```python
from build123d import *

# Parameters (mm, degrees)
SKETCH1_R                  = 6.5
BOSS_EXTRUDE1_DEPTH        = 5
SKETCH2_W                  = 14
SKETCH2_H                  = 5
BOSS_EXTRUDE2_DEPTH        = 50
SKETCH3_R                  = 2.75
CUT_EXTRUDE1_DEPTH         = 115
FILLET2_R                  = 10
CUT_EXTRUDE2_DEPTH         = 74.994932259
CIRPATTERN1_COUNT          = 4
BOSS_EXTRUDE5_START        = -5
BOSS_EXTRUDE5_DEPTH        = 5
FILLET5_R                  = 10
FILLET6_R                  = 10
FLATTEN_BENDS6_START       = -45
FLATTEN_BENDS6_OUTLINE_W   = 14
FLATTEN_BENDS6_OUTLINE_H   = 5
FLATTEN_BENDS6_DEPTH       = 45
FLATTEN_BENDS6_2_DEPTH     = 5
FLATTEN_BENDS6_3_OUTLINE_W = 14
FLATTEN_BENDS6_3_OUTLINE_H = 43.610839391
FLATTEN_BENDS6_3_OUTLINE_R = 2.75
FLATTEN_BENDS6_3_DEPTH     = 5
PROCESS_BENDS6_START       = -94.110839391
PROCESS_BENDS6_OUTLINE_W   = 14
PROCESS_BENDS6_OUTLINE_H   = 5
PROCESS_BENDS6_DEPTH       = 43.610839391
PROCESS_BENDS6_START_2     = 50.5
PROCESS_BENDS6_2_OUTLINE_W = 14
PROCESS_BENDS6_2_OUTLINE_H = 5
PROCESS_BENDS6_2_DEPTH     = 43.610839391
PROCESS_BENDS6_START_3     = -49.958579692
PROCESS_BENDS6_3_OUTLINE_W = 14
PROCESS_BENDS6_3_OUTLINE_H = 45
PROCESS_BENDS6_3_OUTLINE_R = 2.75
PROCESS_BENDS6_3_DEPTH     = 4.458579692
PROCESS_BENDS6_START_4     = 45.5
PROCESS_BENDS6_4_OUTLINE_W = 14
PROCESS_BENDS6_4_OUTLINE_H = 45
PROCESS_BENDS6_4_OUTLINE_R = 2.75
PROCESS_BENDS6_4_DEPTH     = 4.394100308
PROCESS_BENDS6_START_5     = 44.7634
PROCESS_BENDS6_5_OUTLINE_W = 14
PROCESS_BENDS6_5_OUTLINE_H = 45
PROCESS_BENDS6_5_OUTLINE_R = 2.75
PROCESS_BENDS6_5_DEPTH     = 5.7366
PROCESS_BENDS6_START_6     = -50.5
PROCESS_BENDS6_6_OUTLINE_W = 14
PROCESS_BENDS6_6_OUTLINE_H = 45
PROCESS_BENDS6_6_OUTLINE_R = 2.75
PROCESS_BENDS6_6_DEPTH     = 5.7366
PROCESS_BENDS6_START_7     = 5
PROCESS_BENDS6_7_DEPTH     = 14


with BuildPart() as part:
    # Sketch1 → Boss-Extrude1 (new body)
    with BuildSketch(Plane.XY):
        with BuildLine():
            Line((7.22970639, 29.115826375), (7.22970639, 45.5))
            Line((7.22970639, 45.5), (-7.22970639, 45.5))
            Line((-7.22970639, 45.5), (-7.22970639, 29.115826375))
            ThreePointArc((-7.22970639, 29.115826375), (-30, 0), (-7.22970639, -29.115826375))
            Line((-7.22970639, -29.115826375), (-7.22970639, -45.5))
            Line((-7.22970639, -45.5), (7.22970639, -45.5))
            Line((7.22970639, -45.5), (7.22970639, -29.115826375))
            ThreePointArc((7.22970639, -29.115826375), (30, 0), (7.22970639, 29.115826375))
        make_face()
        Circle(SKETCH1_R, mode=Mode.SUBTRACT)
    extrude(amount=BOSS_EXTRUDE1_DEPTH)

    # Sketch2 → Boss-Extrude2 (add)
    with BuildSketch(Plane.XY.offset(5)):
        with Locations((12, 48)):
            Rectangle(SKETCH2_W, SKETCH2_H)
        with Locations((12, -48)):
            Rectangle(SKETCH2_W, SKETCH2_H)
    extrude(amount=-BOSS_EXTRUDE2_DEPTH)

    # Sketch3 → Cut-Extrude1 (cut)
    with BuildSketch(Plane(origin=(0, 50.5, 0), x_dir=(1, 0, 0), z_dir=(0, 1, 0))):
        with Locations(Location((12, 40, 0), (0, 0, 270))):
            Circle(SKETCH3_R)
        with Locations(Location((12, 25, 0), (0, 0, 270))):
            Circle(SKETCH3_R)
    extrude(amount=-CUT_EXTRUDE1_DEPTH, mode=Mode.SUBTRACT)

    # Fillet2
    fillet2_edges = [part.edges().sort_by_distance(p)[0] for p in [
        (7.22970639, -29.115826375, 2.5),
        (-7.22970639, -29.115826375, 2.5),
        (-7.22970639, 29.115826375, 2.5),
        (7.22970639, 29.115826375, 2.5),
    ]]
    fillet(fillet2_edges, radius=FILLET2_R)

    # Sketch4 → Cut-Extrude2 (cut, through all)
    with BuildSketch(Plane(origin=(0, 0, 0), x_dir=(-1, 0, 0), z_dir=(0, 0, -1))):
        with BuildLine():
            Line((-2.993018736, 21.795454545), (-1.496509368, -0.102272727))
            ThreePointArc((-1.496509368, -0.102272727), (0, -1.5), (1.496509368, -0.102272727))
            Line((1.496509368, -0.102272727), (2.993018736, 21.795454545))
            ThreePointArc((2.993018736, 21.795454545), (0, 25), (-2.993018736, 21.795454545))
        make_face()
    cut_extrude2 = extrude(amount=-CUT_EXTRUDE2_DEPTH, mode=Mode.SUBTRACT)

    # CirPattern1: Cut-Extrude2 ×4 about axis
    cirpattern1_axis = Axis((0, 0, 0), (0, 0, 1))
    for i in range(1, CIRPATTERN1_COUNT):
        add(cut_extrude2.rotate(cirpattern1_axis, i * 360 / CIRPATTERN1_COUNT), mode=Mode.SUBTRACT)

    # Sketch41 → Boss-Extrude5 (add)
    with BuildSketch(Plane.XY.offset(5).offset(BOSS_EXTRUDE5_START)):
        with BuildLine():
            Line((7.22970639, 45.5), (19, 45.5))
            Line((19, 45.5), (19, 23.216373532))
            ThreePointArc((19, 23.216373532), (16.077275199, 25.32826923), (12.922279793, 27.074243941))
            ThreePointArc((12.922279793, 27.074243941), (8.771743693, 30.763931751), (7.22970639, 36.098991921))
            Line((7.22970639, 36.098991921), (7.22970639, 45.5))
        make_face()
        with BuildLine():
            Line((19, -45.5), (7.22970639, -45.5))
            Line((7.22970639, -45.5), (7.22970639, -36.098991921))
            ThreePointArc((7.22970639, -36.098991921), (8.771743693, -30.763931751), (12.922279793, -27.074243941))
            ThreePointArc((12.922279793, -27.074243941), (16.077275199, -25.32826923), (19, -23.216373532))
            Line((19, -23.216373532), (19, -45.5))
        make_face()
    extrude(amount=BOSS_EXTRUDE5_DEPTH)

    # Fillet5
    fillet5_edges = [part.edges().sort_by_distance(p)[0] for p in [
        (19, 23.216373532, 2.5),
        (19, -23.216373532, 2.5),
    ]]
    fillet(fillet5_edges, radius=FILLET5_R)

    # Fillet6
    fillet6_edges = [part.edges().sort_by_distance(p)[0] for p in [
        (-7.22970639, 45.5, 2.5),
        (-7.22970639, -45.5, 2.5),
    ]]
    fillet(fillet6_edges, radius=FILLET6_R)

    # Flatten-Bends6: read off the stored shape, not the designer's step
    # Flatten-Bends6 outline → Flatten-Bends6 (cut)
    with BuildSketch(Plane.XY.offset(FLATTEN_BENDS6_START)):
        with Locations((12, 48)):
            Rectangle(FLATTEN_BENDS6_OUTLINE_W, FLATTEN_BENDS6_OUTLINE_H)
        with Locations((12, -48)):
            Rectangle(FLATTEN_BENDS6_OUTLINE_W, FLATTEN_BENDS6_OUTLINE_H)
    extrude(amount=FLATTEN_BENDS6_DEPTH, mode=Mode.SUBTRACT)

    # Flatten-Bends6 2 outline → Flatten-Bends6 2 (cut)
    with BuildSketch(Plane.XY):
        with BuildLine():
            Line((5, 42.2634), (5, 45.5))
            Line((5, 45.5), (2.761321814, 45.5))
            ThreePointArc((2.761321814, 45.5), (2.63064975, 45.499146204), (2.5, 45.496584962))
            Line((2.5, 45.496584962), (2.5, 42.2634))
            Line((2.5, 42.2634), (5, 42.2634))
        make_face()
        with BuildLine():
            Line((5, -45.5), (5, -42.2634))
            Line((5, -42.2634), (2.5, -42.2634))
            Line((2.5, -42.2634), (2.5, -45.496584962))
            ThreePointArc((2.5, -45.496584962), (2.63064975, -45.499146204), (2.761321814, -45.5))
            Line((2.761321814, -45.5), (5, -45.5))
        make_face()
    extrude(amount=FLATTEN_BENDS6_2_DEPTH, mode=Mode.SUBTRACT)

    # Flatten-Bends6 3 outline → Flatten-Bends6 3 (add)
    # profile 1 of 2: a face of its own
    with BuildSketch(Plane.XY):
        with Locations((12, 72.305419696)):
            Rectangle(FLATTEN_BENDS6_3_OUTLINE_W, FLATTEN_BENDS6_3_OUTLINE_H)
        with Locations((12, 74.110839391)):
            Circle(FLATTEN_BENDS6_3_OUTLINE_R, mode=Mode.SUBTRACT)
        with Locations((12, 89.110839391)):
            Circle(FLATTEN_BENDS6_3_OUTLINE_R, mode=Mode.SUBTRACT)
    # profile 2 of 2: a face of its own
    with BuildSketch(Plane.XY):
        with Locations((12, -72.305419696)):
            Rectangle(FLATTEN_BENDS6_3_OUTLINE_W, FLATTEN_BENDS6_3_OUTLINE_H)
        with Locations((12, -89.110839391)):
            Circle(FLATTEN_BENDS6_3_OUTLINE_R, mode=Mode.SUBTRACT)
        with Locations((12, -74.110839391)):
            Circle(FLATTEN_BENDS6_3_OUTLINE_R, mode=Mode.SUBTRACT)
    extrude(amount=FLATTEN_BENDS6_3_DEPTH)

    # Process-Bends6: read off the stored shape, not the designer's step
    # Process-Bends6 outline → Process-Bends6 (cut)
    with BuildSketch(Plane(origin=(0, 0, 0), x_dir=(1, 0, 0), z_dir=(0, 1, 0)).offset(PROCESS_BENDS6_START)):
        with Locations((12, -2.5)):
            Rectangle(PROCESS_BENDS6_OUTLINE_W, PROCESS_BENDS6_OUTLINE_H)
    extrude(amount=PROCESS_BENDS6_DEPTH, mode=Mode.SUBTRACT)

    # Process-Bends6 2 outline → Process-Bends6 2 (cut)
    with BuildSketch(Plane(origin=(0, 0, 0), x_dir=(1, 0, 0), z_dir=(0, 1, 0)).offset(PROCESS_BENDS6_START_2)):
        with Locations((12, -2.5)):
            Rectangle(PROCESS_BENDS6_2_OUTLINE_W, PROCESS_BENDS6_2_OUTLINE_H)
    extrude(amount=PROCESS_BENDS6_2_DEPTH, mode=Mode.SUBTRACT)

    # Process-Bends6 3 outline → Process-Bends6 3 (add)
    with BuildSketch(Plane(origin=(0, 0, 0), x_dir=(1, 0, 0), z_dir=(0, 1, 0)).offset(PROCESS_BENDS6_START_3)):
        with Locations((12, 22.5)):
            Rectangle(PROCESS_BENDS6_3_OUTLINE_W, PROCESS_BENDS6_3_OUTLINE_H)
        with Locations((12, 25)):
            Circle(PROCESS_BENDS6_3_OUTLINE_R, mode=Mode.SUBTRACT)
        with Locations((12, 40)):
            Circle(PROCESS_BENDS6_3_OUTLINE_R, mode=Mode.SUBTRACT)
    extrude(amount=PROCESS_BENDS6_3_DEPTH)

    # Process-Bends6 4 outline → Process-Bends6 4 (add)
    with BuildSketch(Plane(origin=(0, 0, 0), x_dir=(1, 0, 0), z_dir=(0, 1, 0)).offset(PROCESS_BENDS6_START_4)):
        with Locations((12, 22.5)):
            Rectangle(PROCESS_BENDS6_4_OUTLINE_W, PROCESS_BENDS6_4_OUTLINE_H)
        with Locations((12, 25)):
            Circle(PROCESS_BENDS6_4_OUTLINE_R, mode=Mode.SUBTRACT)
        with Locations((12, 40)):
            Circle(PROCESS_BENDS6_4_OUTLINE_R, mode=Mode.SUBTRACT)
    extrude(amount=PROCESS_BENDS6_4_DEPTH)

    # Process-Bends6 5 outline → Process-Bends6 5 (add)
    with BuildSketch(Plane(origin=(0, 0, 0), x_dir=(1, 0, 0), z_dir=(0, 1, 0)).offset(PROCESS_BENDS6_START_5)):
        with Locations((12, 22.5)):
            Rectangle(PROCESS_BENDS6_5_OUTLINE_W, PROCESS_BENDS6_5_OUTLINE_H)
        with Locations((12, 25)):
            Circle(PROCESS_BENDS6_5_OUTLINE_R, mode=Mode.SUBTRACT)
        with Locations((12, 40)):
            Circle(PROCESS_BENDS6_5_OUTLINE_R, mode=Mode.SUBTRACT)
    extrude(amount=PROCESS_BENDS6_5_DEPTH)

    # Process-Bends6 6 outline → Process-Bends6 6 (add)
    with BuildSketch(Plane(origin=(0, 0, 0), x_dir=(1, 0, 0), z_dir=(0, 1, 0)).offset(PROCESS_BENDS6_START_6)):
        with Locations((12, 22.5)):
            Rectangle(PROCESS_BENDS6_6_OUTLINE_W, PROCESS_BENDS6_6_OUTLINE_H)
        with Locations((12, 25)):
            Circle(PROCESS_BENDS6_6_OUTLINE_R, mode=Mode.SUBTRACT)
        with Locations((12, 40)):
            Circle(PROCESS_BENDS6_6_OUTLINE_R, mode=Mode.SUBTRACT)
    extrude(amount=PROCESS_BENDS6_6_DEPTH)

    # Process-Bends6 7 outline → Process-Bends6 7 (cut)
    with BuildSketch(Plane.YZ.offset(PROCESS_BENDS6_START_7)):
        with BuildLine():
            Line((-45.5, -0.7366), (-45.5, -45))
            Line((-45.5, -45), (-44.7634, -45))
            Line((-44.7634, -45), (-44.7634, 0))
            ThreePointArc((-44.7634, 0), (-45.284254855, -0.215745145), (-45.5, -0.7366))
        make_face()
        with BuildLine():
            ThreePointArc((-50.5, -0.7366), (-48.819788761, 3.319788761), (-44.7634, 5))
            Line((-44.7634, 5), (-50.5, 5))
            Line((-50.5, 5), (-50.5, -0.7366))
        make_face()
        with BuildLine():
            ThreePointArc((44.7634, 5), (48.819788761, 3.319788761), (50.5, -0.7366))
            Line((50.5, -0.7366), (50.5, 5))
            Line((50.5, 5), (44.7634, 5))
        make_face()
        with BuildLine():
            Line((45.5, -45), (45.5, -0.7366))
            ThreePointArc((45.5, -0.7366), (45.284254855, -0.215745145), (44.7634, 0))
            Line((44.7634, 0), (44.7634, -45))
            Line((44.7634, -45), (45.5, -45))
        make_face()
    extrude(amount=PROCESS_BENDS6_7_DEPTH, mode=Mode.SUBTRACT)


solid = part.part
```
Input: part model. Units: mm. Frame: model coordinates. A direction names the side the tool comes from. Coordinates: 2 decimals unless noted, no trailing zeros. Write each loop counter-clockwise with the first axis right and the second up, starting at its lowest first coordinate (ties: lowest second). Pieces come first, ordered by that corner, then holes. Notation, with made-up numbers: (-10, 65) -> (-3, 65) arc R3 ccw to (-3, 69) -> close; hole circle Ø3 at (52.5, -4.75). An arc over 180 degrees is marked (long way). Write each question's results on one line, items separated by ' | '.
Item 1: Set-up query: faces 5 (the flat face through (2.5, -44, 2)), 6 (the flat face through (14.111, -2.468, 2.465)), 7 (the flat face through (10.3, -45.5, -22.6)). Return all of +Z, -Z, +X, -X, +Y, -Y with unobstructed straight access to the full face (end or side cutting, diameter ignored); none if empty.
Conclusion:
face 5: +Z, -Z, -Y | face 6: +Z, -Z | face 7: -Z, +X, -X
Item 2: Section query C-C on z = -25. Return loops of the section in (x, y), plus the area to 3 significant figures.
Conclusion:
outline: (5, -50.5) -> (9.25, -50.5) -> (9.25, -45.5) -> (5, -45.5) -> close; (5, 45.5) -> (9.25, 45.5) -> (9.25, 50.5) -> (5, 50.5) -> close; (14.75, -50.5) -> (19, -50.5) -> (19, -45.5) -> (14.75, -45.5) -> close; (14.75, 45.5) -> (19, 45.5) -> (19, 50.5) -> (14.75, 50.5) -> close | area: 85.0 mm^2
Item 3: Section query B-B on y = -10. Return loops of the section in (x, z), plus the area to 3 significant figures.
Conclusion:
outline: (-28.28, 0) -> (-2.19, 0) -> (-2.19, 5) -> (-28.28, 5) -> close; (2.19, 0) -> (28.28, 0) -> (28.28, 5) -> (2.19, 5) -> close | area: 261 mm^2
Item 4: Section query A-A on z = -34.5. Return loops of the section in (x, y).
Conclusion:
outline: (5, -50.5) -> (19, -50.5) -> (19, -45.5) -> (5, -45.5) -> close; (5, 45.5) -> (19, 45.5) -> (19, 50.5) -> (5, 50.5) -> close
Item 5: Material intervals for probe 1 along Z at (x, y) = (12, -48.25); probe 2 along X at (y, z) = (-46.8, -40); probe 3 along Z at (x, y) = (12, -47), sorted ascending.
Conclusion:
probe 1: z = -45 to -42.75, -37.25 to -27.75, -22.25 to 3.82 | probe 2: x = 5 to 9.25, 14.75 to 19 | probe 3: z = -45 to -42.75, -37.25 to -27.75, -22.25 to 4.55
Item 6: Pin query (flat end, axial travel): pin 1 Ø1.2 at (x, z) = (4, 3.5) entering from +Y; pin 2 Ø0.8 at (x, z) = (3.5, 2) entering from -Y; pin 3 Ø3.5 at (x, z) = (12, -25) entering from -Y; pin 4 Ø3.5 at (y, z) = (-43.5, 2) entering from +X. Return the tip coordinate at first contact, or that it passes through.
Conclusion:
pin 1: stops at y = 42.26 | pin 2: stops at y = -42.26 | pin 3: passes through | pin 4: stops at x = 19
Item 7: Mould query, pull axis Z, two halves, no side actions, for faces 1 (the cylindrical face through (11.902, 48.775, 3.364)), 2 (the flat face through (12, 48, -45)), 3 (the cylindrical face through (11.642, 47.965, -42.727)), 4 (the cylindrical face through (30, 0, 2)). Classes: +Z half, -Z half, draft (parallel to the pull), parting line (faces both ways), or undercut.
Conclusion:
face 1: +Z half | face 2: -Z half | face 3: undercut | face 4: draft
Item 8: Section query D-D on x = 12. Count the separate pieces of the cut face and the enclosed holes in it, plus the area to 3 significant figures.
Conclusion:
separate pieces: 6 | enclosed holes: 0 | area: 808 mm^2
